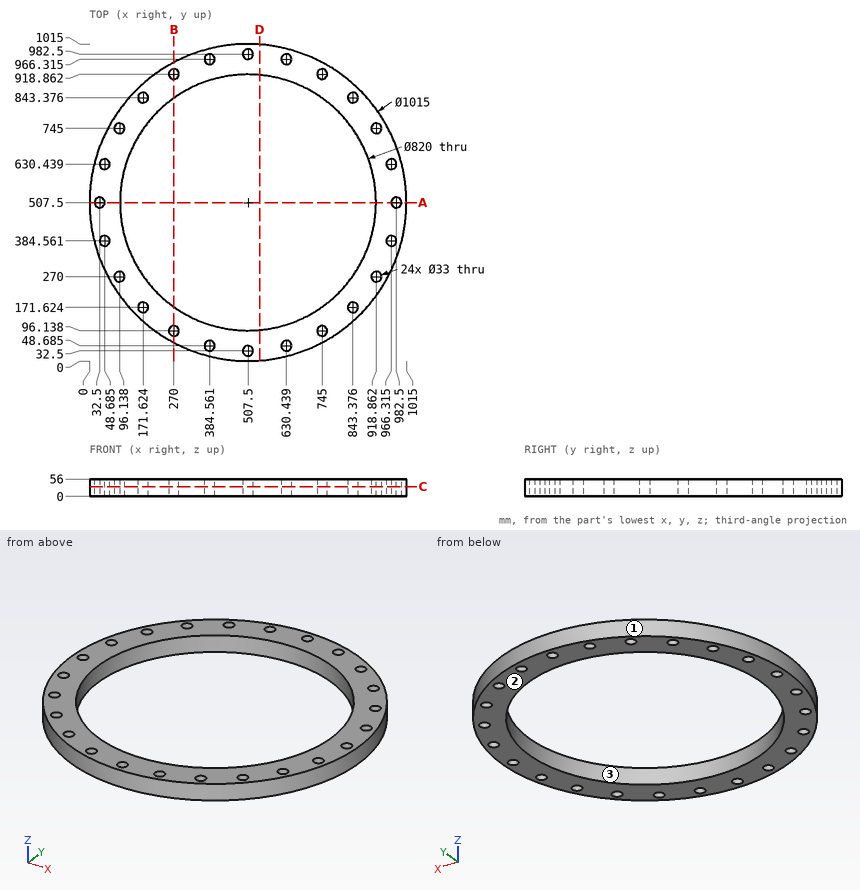
Geometry: see drawing. Coordinates: mm, zero at the bounding-box minimum. Round coordinates to 2 decimals unless told otherwise and drop trailing zeros. Write each loop counter-clockwise with the first axis right and the second up, starting at its lowest first coordinate (ties: lowest second). Pieces come first, ordered by that corner, then holes.
Item 1: Section query A-A (y = 507.5). Return loops of the section in (x, z).
Item 2: Section query C-C (z = 31.5). Give the number of separate pieces and of enclosed holes in the cut face, plus the area to 3 significant figures.
Item 3: Section query D-D (x = 544.5). Return loops of the section in (y, z), plus the area to 3 significant figures.
Item 4: Mould query, pull axis X, two halves, no side actions, for the marked faces 1, 2 and 3. Classes: +X half, -X half, draft (parallel to the pull), parting line (faces both ways), or undercut.
Item 5: Section query B-B (x = 270). Return loops of the section in (y, z).
Item 6: Pin query (flat end, axial travel): P1, Ø10, axis at y = 399, z = 16.5, coming from the +X side; P2, Ø1.5, axis at x = 629.5, z = 45, coming from the -Y side; P3, Ø2, axis at x = 371.5, z = 23.5, coming from the -Y side (1 decimal); P4, Ø2, axis at x = 745, y = 902.5, coming from the +Z side. Return the tip coordinate at first contact, or that it passes through.
Item 7: Material intervals for L1, parallel to X at y = 507, z = 42; L2, parallel to Y at x = 183, z = 35.5 (1 decimal); L3, parallel to Y at x = 747, z = 38 (1 decimal), sorted ascending.
Completed:
1. outline: (0, 0) - (16, 0) - (16, 56) - (0, 56) - close; (49, 0) - (97.5, 0) - (97.5, 56) - (49, 56) - close; (917.5, 0) - (966, 0) - (966, 56) - (917.5, 56) - close; (999, 0) - (1015, 0) - (1015, 56) - (999, 56) - close
2. separate pieces: 1
2. enclosed holes: 25
2. area: 261,000 mm2
3. outline: (1.35, 0) - (99.17, 0) - (99.17, 56) - (1.35, 56) - close; (915.83, 0) - (1013.65, 0) - (1013.65, 56) - (915.83, 56) - close
3. area: 11,000 mm2
4. face 1: parting line
4. face 2: draft
4. face 3: undercut
5. outline: (59, 0) - (79.64, 0) - (79.64, 56) - (59, 56) - close; (112.64, 0) - (173.29, 0) - (173.29, 56) - (112.64, 56) - close; (841.71, 0) - (902.36, 0) - (902.36, 56) - (841.71, 56) - close; (935.36, 0) - (956, 0) - (956, 56) - (935.36, 56) - close
6. P1: stops at x = 1004.33
6. P2: stops at y = 14.7
6. P3: stops at y = 18.3
6. P4: stops at z = 56
7. L1: x = 0 to 16.01, 48.99 to 97.5, 917.5 to 966.01, 998.99 to 1015
7. L2: y = 117.3 to 159.7, 183.6 to 256.9, 758.1 to 831.4, 855.3 to 897.7
7. L3: y = 60.1 to 79.8, 112.5 to 174.7, 840.3 to 902.5, 935.2 to 954.9
